Could you check a few things on this model? Use its own coordinates, in mm. A direction names the side the tool comes from. Round coordinates to 2 decimals unless told otherwise and drop trailing zeros. Loops run counter-clockwise (first coordinate to the right, second up) from the corner with the lowest first, then second, coordinate; pieces in that order, holes last. Notation, with made-up numbers: M -25,51.5 L 2,51.5 A18 cw 2,85.5 Z; hole C -15,-25.5 d8. An arc over 180 degrees is marked long. Answer in a Markdown table with one row per item.
```python
from build123d import *

# Parameters (mm, degrees)
F0_W     = 85
F0_H     = 85
F1_DEPTH = 10
F2_W     = 45
F2_H     = 45
F3_DEPTH = 50
F4_W     = 85
F4_H     = 85
F5_DEPTH = 10
F6_W     = 30
F6_H     = 30
F7_DEPTH = 70


with BuildPart() as f1:
    # F0 (on Top) → F1 (new body)
    with BuildSketch(Plane.XY):
        Rectangle(F0_W, F0_H)
    extrude(amount=F1_DEPTH)

    # F2 (on face) → F3 (join)
    with BuildSketch(Plane.XY.offset(10)):
        Rectangle(F2_W, F2_H)
    extrude(amount=F3_DEPTH)

    # F4 (on face) → F5 (join)
    with BuildSketch(Plane.XY.offset(60)):
        Rectangle(F4_W, F4_H)
    extrude(amount=F5_DEPTH)

    # F6 (on face) → F7 (cut)
    with BuildSketch(Plane.XY.offset(70)):
        Rectangle(F6_W, F6_H)
    extrude(amount=-F7_DEPTH, mode=Mode.SUBTRACT)


solid = f1.part
```
1) I want a section at B-B, the plane x = -35. Please give me the cut outline in (y, z).
Computed:
| item | result |
|---|---|
| outline | M -42.5,0 L 42.5,0 L 42.5,10 L -42.5,10 Z; M -42.5,60 L 42.5,60 L 42.5,70 L -42.5,70 Z |
2) I want a section at D-D, the plane x = -19.5. Please give me the cut outline in (y, z), plus the area to 3 significant figures.
Computed:
| item | result |
|---|---|
| outline | M -42.5,0 L 42.5,0 L 42.5,10 L 22.5,10 L 22.5,60 L 42.5,60 L 42.5,70 L -42.5,70 L -42.5,60 L -22.5,60 L -22.5,10 L -42.5,10 Z |
| area | 3,950 mm² |
3) I need wall thicknesses on line 1 (Y direction, x = -5, z = 15.5); line 2 (Z direction, x = 13.5, y = -30.5). Which ranges of each line are inside material? Lowest first, please.
Computed:
| item | result |
|---|---|
| line 1 | y = -22.5 to -15, 15 to 22.5 |
| line 2 | z = 0 to 10, 60 to 70 |
4) Will these pins go through, and if not, where does the flat tip stop? P1, Ø8, axis at x = 5.5, z = 38.5, coming from the +Y side; P2, Ø1.5, axis at y = 14.5, z = 48, coming from the +X side; P3, Ø9, axis at y = -6.5, z = 19, coming from the -X side.
Computed:
| item | result |
|---|---|
| P1 | stops at y = 22.5 |
| P2 | stops at x = 22.5 |
| P3 | stops at x = -22.5 |
5) Which directions (+Z, -Z, +X, -X, +Y, -Y) give clear straight access to the entire face, cutting with the end or side of a thin tool? Please do faces 1 (the face through (0, -22.5, 35)), 2 (the face through (-15, 0, 35)), 3 (the face through (-29, 1, 10)).
Computed:
| item | result |
|---|---|
| face 1 | +X, -X, -Y |
| face 2 | +Z, -Z |
| face 3 | none |
6) I want a section at C-C, the plane z = 18. Please give me the cut outline in (x, y), plus the area to 4 significant figures.
Computed:
| item | result |
|---|---|
| outline | M -22.5,-22.5 L 22.5,-22.5 L 22.5,22.5 L -22.5,22.5 Z; hole M -15,-15 L 15,-15 L 15,15 L -15,15 Z |
| area | 1,125 mm² |
7) If we mould it in two halves opening along Y, with no side actions, what happens to faces 4 (the face through (0, 15, 35)), 5 (the face through (-1, 42.5, 5)), 6 (the face through (-29, 1, 60)), 7 (the face through (-1, -42.5, 5))? For each: released by +Y, released by -Y, zero draft, split by the parting line, or undercut.
Computed:
| item | result |
|---|---|
| face 4 | undercut |
| face 5 | released by +Y |
| face 6 | zero draft |
| face 7 | released by -Y |
8) I want a section at A-A, the plane y = 9.5. Please give me the cut outline in (x, z), plus the area to 3 significant figures.
Computed:
| item | result |
|---|---|
| outline | M -42.5,0 L -15,0 L -15,70 L -42.5,70 L -42.5,60 L -22.5,60 L -22.5,10 L -42.5,10 Z; M 15,0 L 42.5,0 L 42.5,10 L 22.5,10 L 22.5,60 L 42.5,60 L 42.5,70 L 15,70 Z |
| area | 1,850 mm² |
